CAD build for the part. Positions are in the model's coordinates, mm. A direction names the side the tool comes from. Coordinates: 2 decimals unless noted, no trailing zeros. Order: outer loops, then holes, each group sorted by start corner. A loop starts at its lowest first (then second) coordinate and runs counter-clockwise, first axis right, second up. Notation, with made-up numbers: (12, -38.75) - (40, -38.75) arc R36 cw to (40, 0.25) - close; hole circle Ø1 at (-29, -35.75). An arc over 180 degrees is marked (long way). Return JSON: item names as keys, results as strings.
from build123d import *

# Parameters (mm, degrees)
F0_R     = 12.7
F1_DEPTH = 6.35
F2_R     = 6.35
F3_DEPTH = 6.35
F4_R     = 12.7
F4_R_2   = 6.35
F5_DEPTH = 6.35
F6_R     = 2.54
F7_DEPTH = 19.05
F8_R     = 5.08


with BuildPart() as f1:
    # F0 (on Top) → F1 (new body)
    with BuildSketch(Plane.XY):
        Circle(F0_R)
    extrude(amount=F1_DEPTH)

    # F2 (on face) → F3 (join)
    with BuildSketch(Plane.XY.offset(6.35)):
        Circle(F2_R)
    extrude(amount=F3_DEPTH)

    # F4 (on face) → F5 (join)
    with BuildSketch(Plane.XY.offset(12.7)):
        Circle(F4_R)
        Circle(F4_R_2, mode=Mode.SUBTRACT)
        Circle(F4_R_2)
    extrude(amount=F5_DEPTH)

    # F6 (on face) → F7 (cut)
    with BuildSketch(Plane.XY.offset(19.05)):
        Circle(F6_R)
    extrude(amount=-F7_DEPTH, mode=Mode.SUBTRACT)

    # F8
    f8_edges = [f1.edges().sort_by_distance(p)[0] for p in [
        (-12.7, 0, 12.7),
        (-12.7, 0, 6.35),
    ]]
    fillet(f8_edges, radius=F8_R)


solid = f1.part
Item 1: Band-saw the part on A-A, the plane x = 0. List the corners of the cut face in (y, z).
Findings below:
{"outline": "(-12.7, 0) - (-2.54, 0) - (-2.54, 19.05) - (-12.7, 19.05) - (-12.7, 17.78) arc R5.08 ccw to (-7.62, 12.7) - (-6.35, 12.7) - (-6.35, 6.35) - (-7.62, 6.35) arc R5.08 ccw to (-12.7, 1.27) - close; (2.54, 0) - (12.7, 0) - (12.7, 1.27) arc R5.08 ccw to (7.62, 6.35) - (6.35, 6.35) - (6.35, 12.7) - (7.62, 12.7) arc R5.08 ccw to (12.7, 17.78) - (12.7, 19.05) - (2.54, 19.05) - close"}
Item 2: Which spindle directions (+Z, -Z, +X, -X, +Y, -Y) get a long thin tool onto all of the face, cutting with end or side? Do faces 5 (the cylindrical face through (-0.33, 2.52, 9.66)), 6 (the cylindrical face through (-1.38, -6.2, 9.48)). Say none if no direction does.
Findings below:
{"face 5": "+Z, -Z", "face 6": "none"}
Item 3: Drop flat-ended pins along their axis: P1, Ø1.5, axis at y = -1.5, z = 6, coming from the +X side; P2, Ø1.5, axis at x = 3.5, y = 2.5, coming from the -Z side; P3, Ø6, axis at y = -3, z = 7, coming from the -X side; P4, Ø1.5, axis at x = -3, z = 3, coming from the +Y side. Give the stop position or say it passes through.
Findings below:
{"P1": "stops at x = 10.68", "P2": "stops at z = 0", "P3": "stops at x = -11.63", "P4": "stops at y = 12.31"}
Item 4: Band-saw the part on C-C, the plane z = 10.25. List the corners of the cut face in (x, y).
Findings below:
{"outline": "circle Ø12.7 at (0, 0); hole circle Ø5.08 at (0, 0)"}
Item 5: Mould opens along Z. For faces 1 (the flat face through (3, 0, 19.05)), 2 (the cylindrical face through (-2.75, -12.4, 0.63)), 3 (the flat face through (3, 0, 0)), 4 (the flat face through (-3, 6, 6.35)) say: released by +Z, released by -Z, zero draft, split by the parting line, or undercut.
Findings below:
{"face 1": "released by +Z", "face 2": "zero draft", "face 3": "released by -Z", "face 4": "undercut"}
Item 6: Band-saw the part on D-D, the plane z = 2.25. List the corners of the cut face in (x, y).
Findings below:
{"outline": "circle Ø25.21 at (0, 0); hole circle Ø5.08 at (0, 0)"}
Item 7: Wall check: L1, parallel to Y at x = 0, z = 10.75; L2, parallel to Z at x = -0.5, y = 7.75; L3, parallel to Z at x = 10.5, y = -4.5. Give the ranges that are in metal, low to high. Write a range as [from, to].
Findings below:
{"L1": "y = [-6.35, -2.54], [2.54, 6.35]", "L2": "z = [0, 6.35], [12.7, 19.05]", "L3": "z = [0, 4.64], [14.41, 19.05]"}
